```python
from build123d import *

# Parameters (mm, degrees)
F1_DEPTH       = 20
F3_DEPTH       = 120
F5_DEPTH       = 40
F7_DEPTH       = 160.001
F9_W           = 80
F9_H           = 40
F10_DEPTH      = 159.941314
F10_DEPTH_BACK = 164.311218


with BuildPart() as f1:
    # F0 (on Top) → F1 (new body, symmetric)
    with BuildSketch(Plane.XY):
        with BuildLine():
            Line((0, 50), (0, 15))
            ThreePointArc((0, 15), (4.393398, 4.393398), (15, 0))
            Line((15, 0), (305, 0))
            ThreePointArc((305, 0), (315.606602, 4.393398), (320, 15))
            Line((320, 15), (320, 50))
            Line((320, 50), (260, 50))
            Line((260, 50), (260, 110))
            Line((260, 110), (320, 110))
            Line((320, 110), (320, 145))
            ThreePointArc((320, 145), (315.606602, 155.606602), (305, 160))
            Line((305, 160), (240, 160))
            Line((240, 160), (80, 160))
            Line((80, 160), (15, 160))
            ThreePointArc((15, 160), (4.393398, 155.606602), (0, 145))
            Line((0, 145), (0, 110))
            Line((0, 110), (60, 110))
            Line((60, 110), (60, 50))
            Line((60, 50), (0, 50))
        make_face()
    extrude(amount=F1_DEPTH, both=True)

    # F2 (on face) → F3 (join)
    with BuildSketch(Plane.XY.offset(20)):
        Polygon((240, 160), (160, 160), (80, 160), (160, 0), align=None)
    extrude(amount=F3_DEPTH)

    # F4 (on face) → F5 (join)
    with BuildSketch(Plane.XY):
        Polygon((60, 50), (60, 0), (260, 0), (260, 50), (260, 110), (260, 160), (240, 160), (80, 160), (60, 160), (60, 110), align=None)
    extrude(amount=-F5_DEPTH)

    # F6 (on face) → F7 (cut, through all)
    with BuildSketch(Plane(origin=(0, 160, 0), x_dir=(-1, 0, 0), z_dir=(0, 1, 0))):
        with BuildLine():
            Line((-220, -40), (-100, -40))
            Line((-100, -40), (-100, -15))
            ThreePointArc((-100, -15), (-104.393398, -4.393398), (-115, 0))
            Line((-115, 0), (-205, 0))
            ThreePointArc((-205, 0), (-215.606602, -4.393398), (-220, -15))
            Line((-220, -15), (-220, -40))
        make_face()
    extrude(amount=-F7_DEPTH, mode=Mode.SUBTRACT)

    # F9 (on face) → F10 (cut, two sides)
    with BuildSketch(Plane(origin=(159.88065, -4.368274, 0), x_dir=(0.027312, 0.999627, 0), z_dir=(0.999627, -0.027312, 0))) as f10_sk:
        with Locations((44.369904, 80)):
            Rectangle(F9_W, F9_H)
    extrude(amount=F10_DEPTH, mode=Mode.SUBTRACT)
    extrude(f10_sk.sketch, amount=-F10_DEPTH_BACK, mode=Mode.SUBTRACT)


solid = f1.part
```
Geometry check sheet. Reference: the model listing, model coordinates, mm. A direction names the side the tool comes from. Round coordinates to 2 decimals unless told otherwise and drop trailing zeros. Loops run counter-clockwise (first coordinate to the right, second up) from the corner with the lowest first, then second, coordinate; pieces in that order, holes last. Notation, with made-up numbers: (-20.75, 4.25) -> (0.25, 4.25) arc R27 cw to (0.25, 27.25) -> close; hole circle Ø3 at (47, 85). An arc over 180 degrees is marked (long way). Use a Markdown table: item, result.
(1) Set-up check for faces 1 (the flat face through (30, 25, -20)), 2 (the flat face through (290, 110, 0)), 3 (the flat face through (30, 110, 0)): record each of +Z, -Z, +X, -X, +Y, -Y from which the full face is reachable in a straight line by a thin tool's end or side.
Calculated:
| item | result |
|---|---|
| face 1 | -Z, -X, +Y, -Y |
| face 2 | +Z, -Z, +X |
| face 3 | +Z, -Z, -X |
(2) Scan lines: probe 1 along X at (y, z) = (115, -28.5); probe 2 along Z at (x, y) = (252, 93); probe 3 along Y at (x, z) = (294, -19). Record each from-to range of solid material in increasing order.
Calculated:
| item | result |
|---|---|
| probe 1 | 60 to 100, 220 to 260 |
| probe 2 | -40 to 20 |
| probe 3 | 0 to 50, 110 to 160 |
(3) Mould release check, pull along X, two halves, no side actions. Record for faces 4 (the cylindrical face through (4.51, 155.72, 0.28)), 5 (the flat face through (290, 25, -20)), 6 (the cylindrical face through (104.28, 81.12, -4.51)), 7 (the flat face through (159, 81, 0)): released by +X, released by -X, zero draft, split by the parting line, or undercut.
Calculated:
| item | result |
|---|---|
| face 4 | released by -X |
| face 5 | zero draft |
| face 6 | undercut |
| face 7 | undercut |
(4) Sectioned sample at C-C (x = 86.5). Enter the section's corners in (y, z), then the cut area to 3 significant figures.
Calculated:
| item | result |
|---|---|
| outline | (0, -40) -> (160, -40) -> (160, 140) -> (147, 140) -> (147, 20) -> (0, 20) -> close |
| area | 11,200 mm² |
(5) Sectioned sample at B-B (y = 104.5). Enter the section's corners in (x, z), then the cut area to 3 significant figures.
Calculated:
| item | result |
|---|---|
| outline | (60, -40) -> (100, -40) -> (100, -15) arc R15 cw to (115, 0) -> (205, 0) arc R15 cw to (220, -15) -> (220, -40) -> (260, -40) -> (260, 20) -> (212.25, 20) -> (212.25, 140) -> (107.75, 140) -> (107.75, 20) -> (60, 20) -> close |
| area | 19,800 mm² |
(6) Go/stop test with flat-tipped pins: P1, Ø25, axis at x = 40.5, y = 20.5, coming from the -Z side; P2, Ø12, axis at x = 184, y = 86.5, coming from the -Z side; P3, Ø8, axis at y = 56, z = 26.5, coming from the +X side. Record where each tip stops, or that it passes through.
Calculated:
| item | result |
|---|---|
| P1 | z = -20 |
| P2 | z = 0 |
| P3 | x = 190 |
(7) Sectioned sample at A-A (z = -5). Enter the section's corners in (x, y).
Calculated:
| item | result |
|---|---|
| outline | (0, 15) arc R15 ccw to (15, 0) -> (103.82, 0) -> (103.82, 160) -> (15, 160) arc R15 ccw to (0, 145) -> (0, 110) -> (60, 110) -> (60, 50) -> (0, 50) -> close; (216.18, 0) -> (305, 0) arc R15 ccw to (320, 15) -> (320, 50) -> (260, 50) -> (260, 110) -> (320, 110) -> (320, 145) arc R15 ccw to (305, 160) -> (216.18, 160) -> close |
(8) Sectioned sample at D-D (z = 15). Enter the section's corners in (x, y).
Calculated:
| item | result |
|---|---|
| outline | (0, 15) arc R15 ccw to (15, 0) -> (305, 0) arc R15 ccw to (320, 15) -> (320, 50) -> (260, 50) -> (260, 110) -> (320, 110) -> (320, 145) arc R15 ccw to (305, 160) -> (15, 160) arc R15 ccw to (0, 145) -> (0, 110) -> (60, 110) -> (60, 50) -> (0, 50) -> close |
